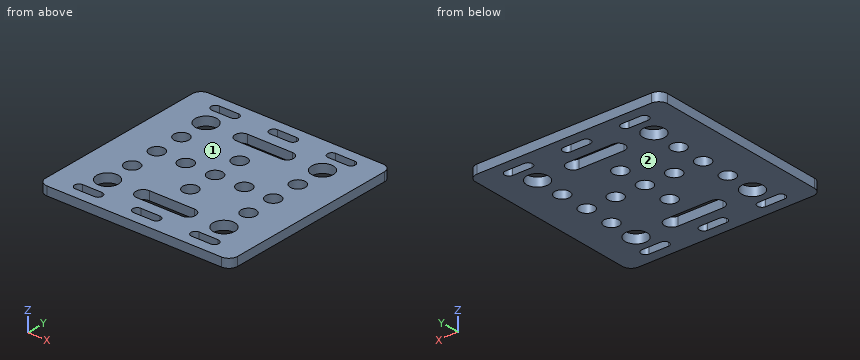
```python
from build123d import *

# Parameters (mm, degrees)
ESQUISSE1_R        = 2.55
ESQUISSE1_R_2      = 3.7
BOSS_EXTRU_1_DEPTH = 3


with BuildPart() as part:
    # Esquisse1 → Boss.-Extru.1 (new body)
    with BuildSketch(Plane.XY):
        with BuildLine():
            Line((101.976699249, 347.427119348), (161.476699249, 347.427119348))
            ThreePointArc((161.476699249, 347.427119348), (163.598019592, 346.548439691), (164.476699249, 344.427119348))
            Line((164.476699249, 344.427119348), (164.476699249, 284.927119348))
            ThreePointArc((164.476699249, 284.927119348), (163.598019592, 282.805799004), (161.476699249, 281.927119348))
            Line((161.476699249, 281.927119348), (101.976699249, 281.927119348))
            ThreePointArc((101.976699249, 281.927119348), (99.855378905, 282.805799004), (98.976699249, 284.927119348))
            Line((98.976699249, 284.927119348), (98.976699249, 344.427119348))
            ThreePointArc((98.976699249, 344.427119348), (99.855378905, 346.548439691), (101.976699249, 347.427119348))
        make_face()
        with Locations((111.877106564, 324.67963586)):
            Circle(ESQUISSE1_R, mode=Mode.SUBTRACT)
        with Locations((131.724446066, 324.67963586)):
            Circle(ESQUISSE1_R, mode=Mode.SUBTRACT)
        with Locations((151.573607548, 324.67963586)):
            Circle(ESQUISSE1_R, mode=Mode.SUBTRACT)
        with Locations((111.876699249, 314.71581075)):
            Circle(ESQUISSE1_R, mode=Mode.SUBTRACT)
        with Locations((131.724446066, 314.71581075)):
            Circle(ESQUISSE1_R, mode=Mode.SUBTRACT)
        with Locations((151.573607548, 314.71581075)):
            Circle(ESQUISSE1_R, mode=Mode.SUBTRACT)
        with Locations((121.727110154, 314.71581075)):
            Circle(ESQUISSE1_R, mode=Mode.SUBTRACT)
        with Locations((141.711298303, 314.71581075)):
            Circle(ESQUISSE1_R, mode=Mode.SUBTRACT)
        with Locations((111.876699249, 304.673954232)):
            Circle(ESQUISSE1_R, mode=Mode.SUBTRACT)
        with Locations((131.724446066, 304.673954232)):
            Circle(ESQUISSE1_R, mode=Mode.SUBTRACT)
        with Locations((151.573607548, 304.673954232)):
            Circle(ESQUISSE1_R, mode=Mode.SUBTRACT)
        with Locations((111.876699249, 334.675400392)):
            Circle(ESQUISSE1_R_2, mode=Mode.SUBTRACT)
        with Locations((151.576699249, 334.675400392)):
            Circle(ESQUISSE1_R_2, mode=Mode.SUBTRACT)
        with Locations((111.876699249, 294.677119348)):
            Circle(ESQUISSE1_R_2, mode=Mode.SUBTRACT)
        with Locations((151.576699249, 294.677119348)):
            Circle(ESQUISSE1_R_2, mode=Mode.SUBTRACT)
        with BuildLine():
            Line((108.630480955, 343.876892887), (115.122917543, 343.876892887))
            ThreePointArc((115.122917543, 343.876892887), (116.622917543, 342.376892887), (115.122917543, 340.876892887))
            Line((115.122917543, 340.876892887), (108.630480955, 340.876892887))
            ThreePointArc((108.630480955, 340.876892887), (107.130480955, 342.376892887), (108.630480955, 343.876892887))
        make_face(mode=Mode.SUBTRACT)
        with BuildLine():
            Line((128.480480955, 343.876892887), (134.972917543, 343.876892887))
            ThreePointArc((134.972917543, 343.876892887), (136.472917543, 342.376892887), (134.972917543, 340.876892887))
            Line((134.972917543, 340.876892887), (128.480480955, 340.876892887))
            ThreePointArc((128.480480955, 340.876892887), (126.980480955, 342.376892887), (128.480480955, 343.876892887))
        make_face(mode=Mode.SUBTRACT)
        with BuildLine():
            Line((148.330480955, 343.876892887), (154.822917543, 343.876892887))
            ThreePointArc((154.822917543, 343.876892887), (156.322917543, 342.376892887), (154.822917543, 340.876892887))
            Line((154.822917543, 340.876892887), (148.330480955, 340.876892887))
            ThreePointArc((148.330480955, 340.876892887), (146.830480955, 342.376892887), (148.330480955, 343.876892887))
        make_face(mode=Mode.SUBTRACT)
        with BuildLine():
            Line((108.630480955, 288.481388741), (115.122917543, 288.481388741))
            ThreePointArc((115.122917543, 288.481388741), (116.622917543, 286.981388741), (115.122917543, 285.481388741))
            Line((115.122917543, 285.481388741), (108.630480955, 285.481388741))
            ThreePointArc((108.630480955, 285.481388741), (107.130480955, 286.981388741), (108.630480955, 288.481388741))
        make_face(mode=Mode.SUBTRACT)
        with BuildLine():
            Line((128.480480955, 288.481388741), (134.972917543, 288.481388741))
            ThreePointArc((134.972917543, 288.481388741), (136.472917543, 286.981388741), (134.972917543, 285.481388741))
            Line((134.972917543, 285.481388741), (128.480480955, 285.481388741))
            ThreePointArc((128.480480955, 285.481388741), (126.980480955, 286.981388741), (128.480480955, 288.481388741))
        make_face(mode=Mode.SUBTRACT)
        with BuildLine():
            Line((148.330480955, 288.481388741), (154.822917543, 288.481388741))
            ThreePointArc((154.822917543, 288.481388741), (156.322917543, 286.981388741), (154.822917543, 285.481388741))
            Line((154.822917543, 285.481388741), (148.330480955, 285.481388741))
            ThreePointArc((148.330480955, 285.481388741), (146.830480955, 286.981388741), (148.330480955, 288.481388741))
        make_face(mode=Mode.SUBTRACT)
        with BuildLine():
            Line((124.031761784, 336.975400392), (139.421636714, 336.975400392))
            ThreePointArc((139.421636714, 336.975400392), (141.721636714, 334.675400392), (139.421636714, 332.375400392))
            Line((139.421636714, 332.375400392), (124.031761784, 332.375400392))
            ThreePointArc((124.031761784, 332.375400392), (121.731761784, 334.675400392), (124.031761784, 336.975400392))
        make_face(mode=Mode.SUBTRACT)
        with BuildLine():
            Line((124.031761784, 297.177119348), (139.421636714, 297.177119348))
            ThreePointArc((139.421636714, 297.177119348), (141.921636714, 294.677119348), (139.421636714, 292.177119348))
            Line((139.421636714, 292.177119348), (124.031761784, 292.177119348))
            ThreePointArc((124.031761784, 292.177119348), (121.531761784, 294.677119348), (124.031761784, 297.177119348))
        make_face(mode=Mode.SUBTRACT)
    extrude(amount=BOSS_EXTRU_1_DEPTH)


solid = part.part
```
Part model, mm, in its own coordinate system. Face numbers are marked on the shaded views. Round coordinates to 2 decimals unless told otherwise and drop trailing zeros.
Item 1: Mould opens along Z. For the marked faces 1 and 2 say: +Z half, -Z half, draft (parallel to the pull), parting line (faces both ways), or undercut.
Item 2: Cut at A-A, the plane x = 111. State how many separate pieces and enclosed holes the cut face has, then the cut area to 3 significant figures.
Item 3: Drill centre lines: line 1 (X direction, y = 287, z = 0.2); line 2 (Y direction, x = 128.5, z = 2.3); line 3 (X direction, y = 292, z = 2.3). Where is each one in solid material? Low to high.
A:
1. face 1: +Z half
1. face 2: -Z half
2. separate pieces: 8
2. enclosed holes: 0
2. area: 92.3 mm2
3. line 1: x = 98.98 to 107.13, 116.62 to 126.98, 136.47 to 146.83, 156.32 to 164.48
3. line 2: y = 281.93 to 285.48, 288.48 to 292.18, 297.18 to 332.38, 336.98 to 340.88, 343.88 to 347.43
3. line 3: x = 98.98 to 109.32, 114.43 to 149.02, 154.13 to 164.48
